The listing builds one solid part. Answer for the finished solid, in the listing's coordinates (mm). A direction names the side the tool comes from. Round coordinates to 2 decimals unless told otherwise and drop trailing zeros. Write each loop counter-clockwise with the first axis right and the second up, starting at its lowest first coordinate (ties: lowest second). Pieces come first, ordered by that corner, then holes.
(1) A cutting plane is placed at A-A, the plane y = 0. Give the vertices of the cut face in (x, z), and give its area (3 significant figures).
(2) Find the intervals of material crossed by probe 1 along Z at (x, y) = (-7.5, 15); probe 2 along X at (y, z) = (18, -109); probe 3 along X at (y, z) = (22, -63), in increasing order.
(3) The mould has two halves that part along X. Classify faces 4 (the face through (-229.993, 0.66, 1.75)), 5 (the face through (229.993, 0.66, -1.75)), 6 (the face through (-150, 0, -145)), 7 (the face through (-3, 0, -125)): +X half, -X half, draft (parallel to the pull), parting line (faces both ways), or undercut.
(4) A cutting plane is placed at B-B, the plane x = -150. Give the vertices of the cut face in (y, z).
(5) A cutting plane is placed at C-C, the plane z = 42.5. Give the vertices of the cut face in (x, y).
(6) For faces 1 (the face through (-139.27, 3.38, 134.86)), 2 (the face through (160.73, 3.38, -134.86)), 3 (the face through (150, 0, 145)), determine the directions among +Z, -Z, +X, -X, +Y, -Y from which every point of the face is accessible in a straight line to the end or side of a thin tool.
(7) Each of these flat-tipped pins is pushed along its axis until it touches: pin 1 Ø4 at (y, z) = (19, -103.5) entering from +X; pin 2 Ø10 at (x, y) = (6, -12) entering from +Z; pin 3 Ø8 at (y, z) = (-22, -44) entering from -X. Where does it stop, or does it pass through?
(8) A cutting plane is placed at D-D, the plane y = 20. Give the vertices of the cut face in (x, z).
from build123d import *

# Parameters (mm, degrees)
SKETCH2_W           = 460
SKETCH2_H           = 60
BOSS_EXTRUDE1_DEPTH = 125
FILLET1_RADIUS      = 30
FILLET1_LENGTH      = 250
FILLET2_RADIUS      = 30
FILLET2_LENGTH      = 250
SKETCH3_R           = 11.25
BOSS_EXTRUDE2_DEPTH = 20


with BuildPart() as part:
    # Sketch2 → Boss-Extrude1 (new, symmetric)
    with BuildSketch(Plane.XY):
        Rectangle(SKETCH2_W, SKETCH2_H)
    extrude(amount=BOSS_EXTRUDE1_DEPTH, both=True)

    # Fillet1: full round fillet: the end face becomes a half cylinder, R = half its width
    fillet1_face = Plane((-230, 0, 0), x_dir=(0, 0, 1), z_dir=(-1, 0, 0))  # on the end face: x along it, z out of the body
    fillet1_slab = fillet1_face.offset(-FILLET1_RADIUS / 2) * Box(FILLET1_LENGTH, 2 * FILLET1_RADIUS, FILLET1_RADIUS, mode=Mode.PRIVATE)  # the body's end, R deep
    fillet1_round = Plane((-200, 0, 0), x_dir=(-1, 0, 0), z_dir=(0, 0, 1)) * Cylinder(FILLET1_RADIUS, FILLET1_LENGTH, mode=Mode.PRIVATE)  # its axis R under the face
    add(fillet1_slab - fillet1_round, mode=Mode.SUBTRACT)

    # Fillet2: full round fillet: the end face becomes a half cylinder, R = half its width
    fillet2_face = Plane((230, 0, 0), x_dir=(0, 0, -1), z_dir=(1, 0, 0))  # on the end face: x along it, z out of the body
    fillet2_slab = fillet2_face.offset(-FILLET2_RADIUS / 2) * Box(FILLET2_LENGTH, 2 * FILLET2_RADIUS, FILLET2_RADIUS, mode=Mode.PRIVATE)  # the body's end, R deep
    fillet2_round = Plane((200, 0, 0), x_dir=(1, 0, 0), z_dir=(0, 0, -1)) * Cylinder(FILLET2_RADIUS, FILLET2_LENGTH, mode=Mode.PRIVATE)  # its axis R under the face
    add(fillet2_slab - fillet2_round, mode=Mode.SUBTRACT)

    # Sketch3 → Boss-Extrude2 (add)
    with BuildSketch(Plane.XY.offset(125)):
        with Locations((-150, 0)):
            Circle(SKETCH3_R)
        with Locations((150, 0)):
            Circle(SKETCH3_R)
    boss_extrude2 = extrude(amount=BOSS_EXTRUDE2_DEPTH)

    # Mirror1: Boss-Extrude2 across plane
    add(boss_extrude2.mirror(Plane.XY))


solid = part.part
Solutions:
1. outline: (-230, -125) - (-161.25, -125) - (-161.25, -145) - (-138.75, -145) - (-138.75, -125) - (138.75, -125) - (138.75, -145) - (161.25, -145) - (161.25, -125) - (230, -125) - (230, 125) - (161.25, 125) - (161.25, 145) - (138.75, 145) - (138.75, 125) - (-138.75, 125) - (-138.75, 145) - (-161.25, 145) - (-161.25, 125) - (-230, 125) - close
1. area: 117,000 mm2
2. probe 1: z = -125 to 125
2. probe 2: x = -224 to 224
2. probe 3: x = -220.4 to 220.4
3. face 4: -X half
3. face 5: +X half
3. face 6: draft
3. face 7: undercut
4. outline: (-30, -125) - (-11.25, -125) - (-11.25, -145) - (11.25, -145) - (11.25, -125) - (30, -125) - (30, 125) - (11.25, 125) - (11.25, 145) - (-11.25, 145) - (-11.25, 125) - (-30, 125) - close
5. outline: (-200, -30) - (200, -30) arc R30 ccw to (200, 30) - (-200, 30) arc R30 ccw to start
6. face 1: +Z
6. face 2: -Z
6. face 3: +Z, +X, -X, +Y, -Y
7. pin 1: stops at x = 224.72
7. pin 2: stops at z = 125
7. pin 3: stops at x = -224
8. outline: (-222.36, -125) - (222.36, -125) - (222.36, 125) - (-222.36, 125) - close
